Read the model definition and answer for the solid it produces. Units are mm, in the model's axes. A direction names the side the tool comes from. Round coordinates to 2 decimals unless told otherwise and drop trailing zeros. Write each loop counter-clockwise with the first axis right and the second up, starting at its lowest first coordinate (ties: lowest second). Pieces come first, ordered by that corner, then holes. Notation, with made-up numbers: (67, 25) - (78, 25) arc R29 ccw to (78, 58) - close; hole circle Ø9 at (53, 2). An arc over 180 degrees is marked (long way). Answer as CSV lines item,"result". Start each with the question number.
1) For a pull along Z with two mould halves and no side action, classify faces 4 (the flat face through (3, -3, 0)), 5 (the flat face through (0.81, -2.96, -3.81)), 6 (the flat face through (0, -3, 3.5)) as +Z half, -Z half, draft (parallel to the pull), parting line (faces both ways), or undercut.
2) Find section B-B on y = -1.85. Determine the outline of the cut face in (x, z), then the cut area to 3 significant figures.
3) Find section A-A on z = -3.5. Determine the outline of the cut face in (x, y), then the cut area to 3 significant figures.
4) Each of these flat-tipped pins is pushed along its axis until it touches: pin 1 (0.5 mm diameter, centred on y = -2, z = -3.5, fed in from +X); pin 2 (1.5 mm diameter, centred on y = -4, z = 0.5, fed in from +X); pin 3 (0.8 mm diameter, centred on y = -4, z = -3.5, fed in from -X). Where does it stop, or does it pass through?
5) Consider line 1 along Z through (x, y) = (0, -5.25); line 2 along X through (y, z) = (-1.2, -5); line 3 along X through (y, z) = (-3.25, 0.25). Determine where each line is inside the solid, lowest interval first.
6) Find section D-D on z = -5. Determine the outline of the cut face in (x, y).
7) Find section C-C on x = 0. Determine the outline of the cut face in (y, z).
8) Which of the six approach directions +Z, -Z, +X, -X, +Y, -Y give full straight-line access (tool end or side, diameter ignored) to faces 1 (the flat face through (-3, -3, 0)), 2 (the flat face through (3.5, -3, -3)), 3 (the flat face through (3.5, -3, 2.5))?
from build123d import *

# Parameters (mm, degrees)
F1_DEPTH = 6


with BuildPart() as f1:
    # F0 (on Front) → F1 (new body)
    with BuildSketch(Plane.XZ):
        with BuildLine():
            Line((4, 3.5), (-4, 3.5))
            Line((-4, 3.5), (-4, 2.5))
            Line((-4, 2.5), (-3, 2.5))
            Line((-3, 2.5), (-3, -2.5))
            Line((-3, -2.5), (-3.5, -2.5))
            Line((-3.5, -2.5), (-3.5, -4.038462))
            Line((-3.5, -4.038462), (-2.7, -6.5))
            Line((-2.7, -6.5), (-1.25, -6.5))
            Line((-1.25, -6.5), (-0.381107, -1.190486))
            ThreePointArc((-0.381107, -1.190486), (-0.736925, 1.009674), (1.25, 0))
            ThreePointArc((1.25, 0), (1.009674, -0.736925), (0.381107, -1.190486))
            Line((0.381107, -1.190486), (1.25, -6.5))
            Line((1.25, -6.5), (2.7, -6.5))
            Line((2.7, -6.5), (3.5, -4.038462))
            Line((3.5, -4.038462), (3.5, -2.5))
            Line((3.5, -2.5), (3, -2.5))
            Line((3, -2.5), (3, 2.5))
            Line((3, 2.5), (4, 2.5))
            Line((4, 2.5), (4, 3.5))
        make_face()
    extrude(amount=F1_DEPTH)


solid = f1.part
Check values:
1,face 4,"undercut"
1,face 5,"-Z half"
1,face 6,"+Z half"
2,outline,"(-4, 2.5) - (-3, 2.5) - (-3, -2.5) - (-3.5, -2.5) - (-3.5, -4.04) - (-2.7, -6.5) - (-1.25, -6.5) - (-0.38, -1.19) arc R1.25 cw (long way) to (0.38, -1.19) - (1.25, -6.5) - (2.7, -6.5) - (3.5, -4.04) - (3.5, -2.5) - (3, -2.5) - (3, 2.5) - (4, 2.5) - (4, 3.5) - (-4, 3.5) - close"
2,area,"50.5 mm^2"
3,outline,"(-3.5, -6) - (-0.76, -6) - (-0.76, 0) - (-3.5, 0) - close; (0.76, -6) - (3.5, -6) - (3.5, 0) - (0.76, 0) - close"
3,area,"32.9 mm^2"
4,pin 1,"stops at x = 3.5"
4,pin 2,"stops at x = 3"
4,pin 3,"stops at x = -3.5"
5,line 1,"z = 1.25 to 3.5"
5,line 2,"x = -3.19 to -1, 1 to 3.19"
5,line 3,"x = -3 to -1.22, 1.22 to 3"
6,outline,"(-3.19, -6) - (-1, -6) - (-1, 0) - (-3.19, 0) - close; (1, -6) - (3.19, -6) - (3.19, 0) - (1, 0) - close"
7,outline,"(-6, 1.25) - (0, 1.25) - (0, 3.5) - (-6, 3.5) - close"
8,face 1,"-X, +Y, -Y"
8,face 2,"-Z, +X, +Y, -Y"
8,face 3,"+X, +Y, -Y"
